The listing builds one solid part. Answer for the finished solid, in the listing's coordinates (mm). Round coordinates to 2 decimals unless told otherwise and drop trailing zeros. Write each loop counter-clockwise with the first axis right and the second up, starting at its lowest first coordinate (ties: lowest second). Pieces come first, ordered by that corner, then holes. Notation, with made-up numbers: (-3, 16.25) - (49, 16.25) arc R17 cw to (49, 38.25) - close; hole circle Ø4 at (-39.75, 35.25). An arc over 180 degrees is marked (long way). Return JSON: item names as keys, results as strings. Group by question number.
(1) Section C-C, the plane x = 11.75 is taken. Write down the section's boundary in (y, z), then the cut area to 3 significant figures.
(2) Section D-D, the plane x = -35 is taken. Write down the section's boundary in (y, z).
(3) Section B-B, the plane z = -27.5 is taken. Write down the section's boundary in (x, y), then the cut area to 3 significant figures.
(4) Section A-A, the plane y = -95 is taken. Write down the section's boundary in (x, z).
(5) Each of these flat-tipped pins is pushed along its axis until it touches: pin 1 (9.5 mm diameter, centred on x = 11.75, z = -27.5, fed in from -Y); pin 2 (5 mm diameter, centred on x = -14.5, z = -30.5, fed in from -Y); pin 3 (12 mm diameter, centred on x = 24.5, y = -68, fed in from -Z); pin 4 (23.5 mm diameter, centred on x = 12.5, z = -23, fed in from -Y). Where does it stop, or does it pass through?
(6) Find the intervals of material crossed by line 1 along Z through (x, y) = (7, -2); line 2 along Z through (x, y) = (-37, -3.5); line 3 along Y through (x, z) = (26.5, 6), in increasing order. Write a range as [from, to].
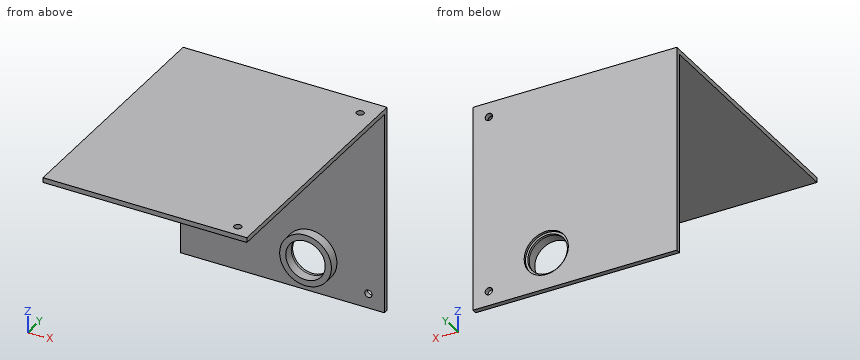
```python
from build123d import *

# Parameters (mm, degrees)
SKETCH1_W               = 83.5
SKETCH1_H               = 85
BOSS_EXTRUDE1_DEPTH     = 2
SKETCH2_W               = 83.5
SKETCH2_H               = 2
BOSS_EXTRUDE2_DEPTH     = 100
SKETCH3_R               = 8.1
SKETCH3_R_2             = 10.6
BOSS_EXTRUDE3_DEPTH     = 4
SKETCH3_3_R             = 8.1
CUT_EXTRUDE3_DEPTH      = 101
CUT_EXTRUDE3_DEPTH_BACK = 3
SKETCH4_R               = 9.05
CUT_EXTRUDE4_DEPTH      = 1
CUT_EXTRUDE5_REACH      = 87
SKETCH5_R               = 1.5
CUT_EXTRUDE6_REACH      = 104
SKETCH6_R               = 1.5


with BuildPart() as part:
    # Sketch1 → Boss-Extrude1 (new body)
    with BuildSketch(Plane(origin=(0, 0, 0), x_dir=(1, 0, 0), z_dir=(0, 1, 0))):
        Rectangle(SKETCH1_W, SKETCH1_H)
    extrude(amount=BOSS_EXTRUDE1_DEPTH)

    # Sketch2 → Boss-Extrude2 (add)
    with BuildSketch(Plane(origin=(0, 0, 0), x_dir=(-1, 0, 0), z_dir=(0, -1, 0))):
        with Locations((0, -41.5)):
            Rectangle(SKETCH2_W, SKETCH2_H)
    extrude(amount=BOSS_EXTRUDE2_DEPTH)

    # Sketch3 → Boss-Extrude3 (add)
    with BuildSketch(Plane(origin=(0, 0, 0), x_dir=(-1, 0, 0), z_dir=(0, -1, 0))):
        with Locations((-11.75, 27.5)):
            Circle(SKETCH3_R)
        with Locations((-11.75, 27.5)):
            Circle(SKETCH3_R_2)
        with Locations((-11.75, 27.5)):
            Circle(SKETCH3_R, mode=Mode.SUBTRACT)
    extrude(amount=BOSS_EXTRUDE3_DEPTH)

    # Sketch3<3> → Cut-Extrude3 (cut, two sides)
    with BuildSketch(Plane(origin=(0, 0, 0), x_dir=(-1, 0, 0), z_dir=(0, -1, 0))) as cut_extrude3_sk:
        with Locations((-11.75, 27.5)):
            Circle(SKETCH3_3_R)
    extrude(amount=CUT_EXTRUDE3_DEPTH, mode=Mode.SUBTRACT)
    extrude(cut_extrude3_sk.sketch, amount=-CUT_EXTRUDE3_DEPTH_BACK, mode=Mode.SUBTRACT)

    # Sketch4 → Cut-Extrude4 (cut)
    with BuildSketch(Plane(origin=(0, 2, 0), x_dir=(1, 0, 0), z_dir=(0, 1, 0))):
        with Locations((11.75, 27.5)):
            Circle(SKETCH4_R)
    extrude(amount=-CUT_EXTRUDE4_DEPTH, mode=Mode.SUBTRACT)

    # Sketch5 → Cut-Extrude5 (cut, up to next)
    with BuildSketch(Plane.XY.offset(42.5), mode=Mode.PRIVATE) as cut_extrude5_sk1:
        with Locations((35.25, -95)):
            Circle(SKETCH5_R)
    cut_extrude5_tool1 = extrude(cut_extrude5_sk1.sketch, amount=-CUT_EXTRUDE5_REACH, mode=Mode.PRIVATE) & part.part
    add(cut_extrude5_tool1.solids().sort_by_distance((35.25, -95, 42.5))[0], mode=Mode.SUBTRACT)
    # Sketch5 → Cut-Extrude5 (cut, up to next)
    with BuildSketch(Plane.XY.offset(42.5), mode=Mode.PRIVATE) as cut_extrude5_sk2:
        with Locations((35.25, -6)):
            Circle(SKETCH5_R)
    cut_extrude5_tool2 = extrude(cut_extrude5_sk2.sketch, amount=-CUT_EXTRUDE5_REACH, mode=Mode.PRIVATE) & part.part
    add(cut_extrude5_tool2.solids().sort_by_distance((35.25, -6, 42.5))[0], mode=Mode.SUBTRACT)

    # Sketch6 → Cut-Extrude6 (cut, up to next)
    with BuildSketch(Plane(origin=(0, 2, 0), x_dir=(1, 0, 0), z_dir=(0, 1, 0)), mode=Mode.PRIVATE) as cut_extrude6_sk1:
        with Locations((35.25, -36.5)):
            Circle(SKETCH6_R)
    cut_extrude6_tool1 = extrude(cut_extrude6_sk1.sketch, amount=-CUT_EXTRUDE6_REACH, mode=Mode.PRIVATE) & part.part
    add(cut_extrude6_tool1.solids().sort_by_distance((35.25, 2, 36.5))[0], mode=Mode.SUBTRACT)
    # Sketch6 → Cut-Extrude6 (cut, up to next)
    with BuildSketch(Plane(origin=(0, 2, 0), x_dir=(1, 0, 0), z_dir=(0, 1, 0)), mode=Mode.PRIVATE) as cut_extrude6_sk2:
        with Locations((35.25, 36.5)):
            Circle(SKETCH6_R)
    cut_extrude6_tool2 = extrude(cut_extrude6_sk2.sketch, amount=-CUT_EXTRUDE6_REACH, mode=Mode.PRIVATE) & part.part
    add(cut_extrude6_tool2.solids().sort_by_distance((35.25, 2, -36.5))[0], mode=Mode.SUBTRACT)


solid = part.part
```
Working result:
{
 "1": {"outline": "(-100, 40.5) - (0, 40.5) - (0, -16.9) - (-4, -16.9) - (-4, -19.4) - (1, -19.4) - (1, -18.45) - (2, -18.45) - (2, 42.5) - (-100, 42.5) - close; (-4, -38.1) - (0, -38.1) - (0, -42.5) - (2, -42.5) - (2, -36.55) - (1, -36.55) - (1, -35.6) - (-4, -35.6) - close", "area": "356 mm^2"},
 "2": {"outline": "(-100, 40.5) - (0, 40.5) - (0, -42.5) - (2, -42.5) - (2, 42.5) - (-100, 42.5) - close"},
 "3": {"outline": "(-41.75, 0) - (1.15, 0) - (1.15, -4) - (3.65, -4) - (3.65, 1) - (2.7, 1) - (2.7, 2) - (-41.75, 2) - close; (19.85, -4) - (22.35, -4) - (22.35, 0) - (41.75, 0) - (41.75, 2) - (20.8, 2) - (20.8, 1) - (19.85, 1) - close", "area": "153 mm^2"},
 "4": {"outline": "(-41.75, 40.5) - (33.75, 40.5) - (33.75, 42.5) - (-41.75, 42.5) - close; (36.75, 40.5) - (41.75, 40.5) - (41.75, 42.5) - (36.75, 42.5) - close"},
 "5": {"pin 1": "passes through", "pin 2": "stops at y = 0", "pin 3": "stops at z = 40.5", "pin 4": "stops at y = -4"},
 "6": {"line 1": "z = [-36.98, -34.06], [-20.94, -18.02], [40.5, 42.5]", "line 2": "z = [40.5, 42.5]", "line 3": "y = [0, 2]"}
}
